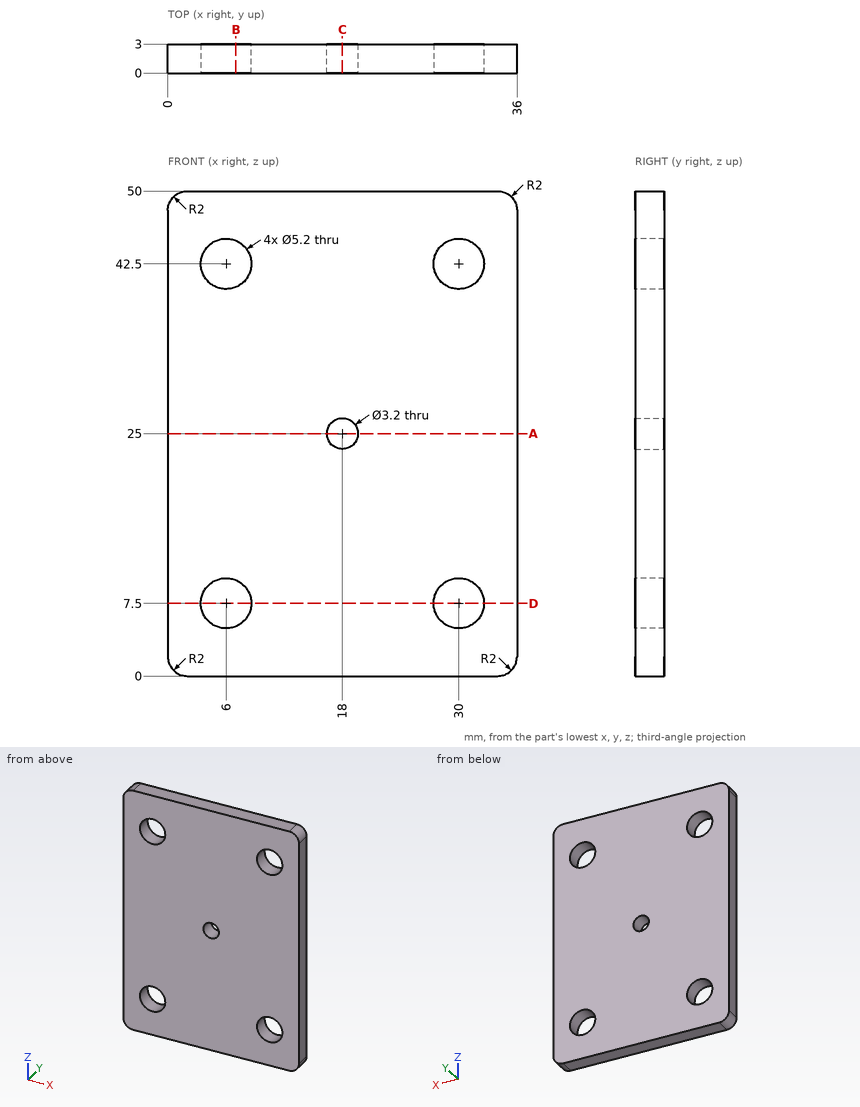
Drawing for the job (mm, zero at the part's lowest x, y, z). Coordinates: 2 decimals unless noted, no trailing zeros. Order: outer loops, then holes, each group sorted by start corner. A loop starts at its lowest first (then second) coordinate and runs counter-clockwise, first axis right, second up. Notation, with made-up numbers: (1, 4.5) -> (56, 4.5) arc R26 cw to (56, 41.5) -> close; hole circle Ø8 at (3, -3). An arc over 180 degrees is marked (long way). Answer in a Markdown table with one row per item.
1) Band-saw the part on D-D (z = 7.5). List the corners of the cut face in (x, y), and give its area (3 significant figures).
Check values:
| item | result |
|---|---|
| outline | (0, 0) -> (3.4, 0) -> (3.4, 3) -> (0, 3) -> close; (8.6, 0) -> (27.4, 0) -> (27.4, 3) -> (8.6, 3) -> close; (32.6, 0) -> (36, 0) -> (36, 3) -> (32.6, 3) -> close |
| area | 76.8 mm2 |
2) Band-saw the part on C-C (x = 18). List the corners of the cut face in (y, z), and give its area (3 significant figures).
Check values:
| item | result |
|---|---|
| outline | (0, 0) -> (3, 0) -> (3, 23.4) -> (0, 23.4) -> close; (0, 26.6) -> (3, 26.6) -> (3, 50) -> (0, 50) -> close |
| area | 140 mm2 |
3) Band-saw the part on B-B (x = 7). List the corners of the cut face in (y, z).
Check values:
| item | result |
|---|---|
| outline | (0, 0) -> (3, 0) -> (3, 5.1) -> (0, 5.1) -> close; (0, 9.9) -> (3, 9.9) -> (3, 40.1) -> (0, 40.1) -> close; (0, 44.9) -> (3, 44.9) -> (3, 50) -> (0, 50) -> close |
4) Band-saw the part on A-A (z = 25). List the corners of the cut face in (x, y).
Check values:
| item | result |
|---|---|
| outline | (0, 0) -> (16.4, 0) -> (16.4, 3) -> (0, 3) -> close; (19.6, 0) -> (36, 0) -> (36, 3) -> (19.6, 3) -> close |
5) Drill centre lines: line 1 (Z direction, x = 6, y = 1.2); line 2 (X direction, y = 1.35, z = 7.5); line 3 (X direction, y = 2.25, z = 25). Where is each one in solid material? Low to high.
Check values:
| item | result |
|---|---|
| line 1 | 0 to 4.9, 10.1 to 39.9, 45.1 to 50 |
| line 2 | 0 to 3.4, 8.6 to 27.4, 32.6 to 36 |
| line 3 | 0 to 16.4, 19.6 to 36 |
